Answer from the drawing. Dimensions are ordinates in mm from the lowest x, y and z of the part. Give positions to 0.01 mm unless a question says otherwise; leave off trailing zeros. Loops run counter-clockwise (first coordinate to the right, second up) from the corner with the lowest first, then second, coordinate; pieces in that order, holes last. Notation, with made-up numbers: M 35,85.25 L 66,85.25 A16 cw 66,99.25 Z; hole C -33,34 d9. An arc over 180 degrees is marked long. Return JSON: item names as keys, results as strings. Group by question number.
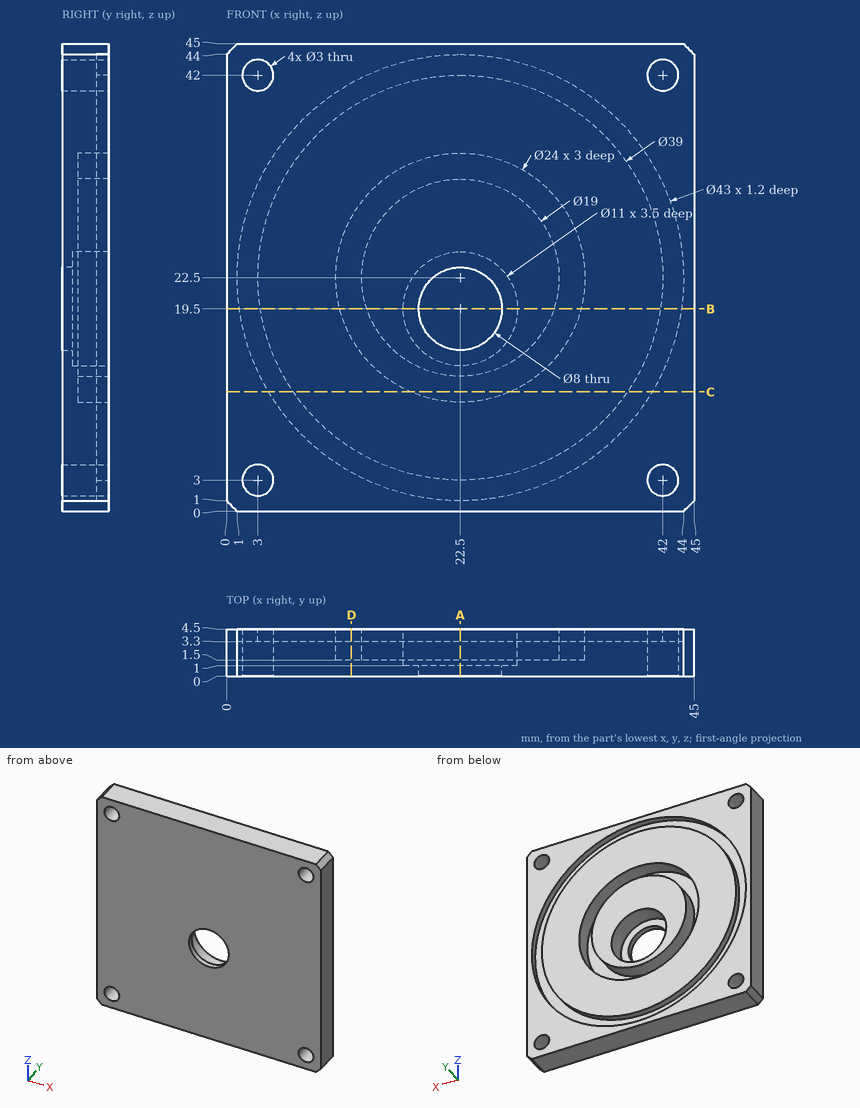
1. Find section A-A (x = 22.5). Write down the section's boundary in (y, z), and give its area (3 significant figures).
2. Find section D-D (x = 12). Write down the section's boundary in (y, z).
3. Find section B-B (z = 19.5). Write down the section's boundary in (x, y), and give its area (3 significant figures).
4. Straight lines are drawn through the part: line 1 along X through (y, z) = (0.9, 3); line 2 along Z through (x, y) = (7, 4.15); line 3 along X through (y, z) = (0.6, 19.5). For each, find the intervals that lie inside material, in ascending order.
5. A flat-ended cylindrical pin translates along its axis: P1, Ø1.5, axis at x = 7.5, z = 6.5, coming from the -Y side. Find the tip coordinate at first contact, or state that the pin passes through.
6. Find section C-C (z = 11.5). Write down the section's boundary in (x, y).
Result:
{
 "1": {"outline": "M 0,0 L 4.5,0 L 4.5,1 L 3.3,1 L 3.3,3 L 4.5,3 L 4.5,10.5 L 1.5,10.5 L 1.5,13 L 4.5,13 L 4.5,14 L 1,14 L 1,15.5 L 0,15.5 Z; M 0,23.5 L 1,23.5 L 1,25 L 4.5,25 L 4.5,32 L 1.5,32 L 1.5,34.5 L 4.5,34.5 L 4.5,42 L 3.3,42 L 3.3,44 L 4.5,44 L 4.5,45 L 0,45 Z", "area": "136 mm2"},
 "2": {"outline": "M 0,0 L 4.5,0 L 4.5,3.74 L 3.3,3.74 L 3.3,6.07 L 4.5,6.07 L 4.5,16.69 L 1.5,16.69 L 1.5,28.31 L 4.5,28.31 L 4.5,38.93 L 3.3,38.93 L 3.3,41.26 L 4.5,41.26 L 4.5,45 L 0,45 Z"},
 "3": {"outline": "M 0,0 L 18.5,0 L 18.5,1 L 17,1 L 17,4.5 L 13.49,4.5 L 13.49,1.5 L 10.88,1.5 L 10.88,4.5 L 3.23,4.5 L 3.23,3.3 L 1.21,3.3 L 1.21,4.5 L 0,4.5 Z; M 26.5,0 L 45,0 L 45,4.5 L 43.79,4.5 L 43.79,3.3 L 41.77,3.3 L 41.77,4.5 L 34.12,4.5 L 34.12,1.5 L 31.51,1.5 L 31.51,4.5 L 28,4.5 L 28,1 L 26.5,1 Z", "area": "136 mm2"},
 "4": {"line 1": "x = 0 to 1.5, 4.5 to 40.5, 43.5 to 45", "line 2": "z = 0 to 7.6, 10.67 to 34.33, 37.4 to 45", "line 3": "x = 0 to 18.5, 26.5 to 45"},
 "5": {"P1": "stops at y = 0"},
 "6": {"outline": "M 0,0 L 45,0 L 45,4.5 L 40.97,4.5 L 40.97,3.3 L 38.6,3.3 L 38.6,4.5 L 27.3,4.5 L 27.3,1.5 L 17.7,1.5 L 17.7,4.5 L 6.4,4.5 L 6.4,3.3 L 4.03,3.3 L 4.03,4.5 L 0,4.5 Z"}
}
